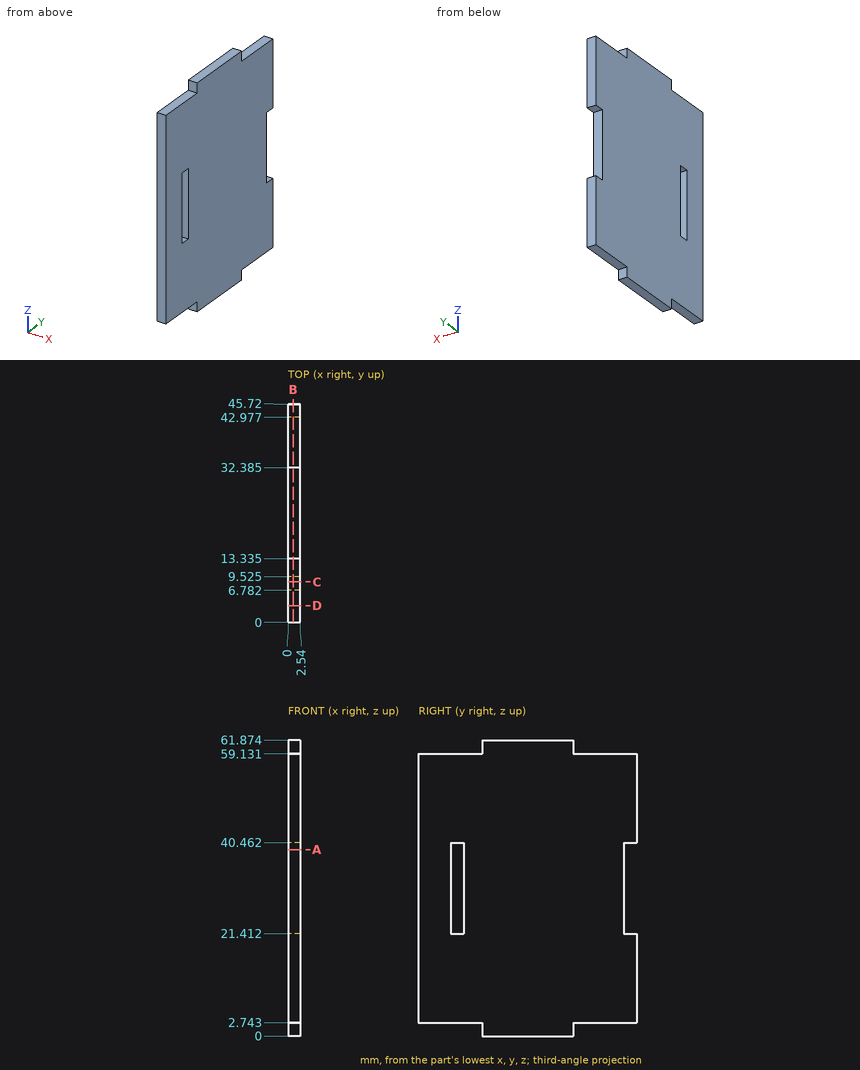
Geometry check sheet. Reference: drawing and pictorial views, mm from the part's lowest x, y, z. Coordinates: 2 decimals unless noted, no trailing zeros. Order: outer loops, then holes, each group sorted by start corner. A loop starts at its lowest first (then second) coordinate and runs counter-clockwise, first axis right, second up. Notation, with made-up numbers: M 22,33.25 L 71,33.25 A12 ccw 71,39.25 Z; hole C 47.5,-16.5 d8. An arc over 180 degrees is marked long. Write each question's results on one line, items separated by ' | '. Start each with the question number.
1. Cross-section at C-C on y = 8.5. Record the cut outline in (x, z).
2. Cross-section at D-D on y = 3.5. Record the cut outline in (x, z).
3. Cross-section at A-A on z = 39. Record the cut outline in (x, y) (1 decimal), and give its area (3 significant figures).
4. Cross-section at B-B on x = 1.05. Record the cut outline in (y, z) (1 decimal).
5. Material ranges on probe 1 along Y at (x, z) = (1.8, 33) (1 decimal); probe 2 along Z at (x, y) = (1.8, 40), recorded low to high.
6. Go/stop test with flat-tipped pins: P1, Ø1.3, axis at x = 1, y = 40, coming from the +Z side; P2, Ø0.8, axis at x = 1.5, z = 61, coming from the -Y side (3 decimals); P3, Ø0.8, axis at x = 1.5, z = 2, coming from the +Y side (3 decimals). Record where each tip stops, or that it passes through.
Checks:
1) outline: M 0,2.74 L 2.54,2.74 L 2.54,21.41 L 0,21.41 Z; M 0,40.46 L 2.54,40.46 L 2.54,59.13 L 0,59.13 Z
2) outline: M 0,2.74 L 2.54,2.74 L 2.54,59.13 L 0,59.13 Z
3) outline: M 0,0 L 2.5,0 L 2.5,6.8 L 0,6.8 Z; M 0,9.5 L 2.5,9.5 L 2.5,43 L 0,43 Z | area: 102 mm²
4) outline: M 0,2.7 L 13.3,2.7 L 13.3,0 L 32.4,0 L 32.4,2.7 L 45.7,2.7 L 45.7,21.4 L 43,21.4 L 43,40.5 L 45.7,40.5 L 45.7,59.1 L 32.4,59.1 L 32.4,61.9 L 13.3,61.9 L 13.3,59.1 L 0,59.1 Z; hole M 6.8,21.4 L 9.5,21.4 L 9.5,40.5 L 6.8,40.5 Z
5) probe 1: y = 0 to 6.8, 9.5 to 43 | probe 2: z = 2.74 to 59.13
6) P1: stops at z = 59.13 | P2: stops at y = 13.335 | P3: stops at y = 32.385
